```python
from build123d import *

# Parameters (mm, degrees)
F0_W     = 75
F0_H     = 70
F0_R     = 5
F0_R_2   = 2
F1_DEPTH = 2
F2_DEPTH = 7


with BuildPart() as f1:
    # F0 (on Top) → F1 (new body)
    with BuildSketch(Plane.XY):
        with Locations((4.717057, 0)):
            Rectangle(F0_W, F0_H)
        with Locations((4.717057, 0)):
            Circle(F0_R, mode=Mode.SUBTRACT)
        with Locations((34.717057, 0)):
            Circle(F0_R_2, mode=Mode.SUBTRACT)
    extrude(amount=F1_DEPTH)

    # F0 (on Top) → F2 (join)
    with BuildSketch(Plane.XY):
        with Locations((4.717057, 0)):
            Circle(F0_R)
        with Locations((34.717057, 0)):
            Circle(F0_R_2)
    extrude(amount=F2_DEPTH)


solid = f1.part
```
Can you work these out from the model? Positions are in its coordinate system, mm. A direction names the side the tool comes from. Give positions to 0.01 mm unless a question says otherwise; leave off trailing zeros. Loops run counter-clockwise (first coordinate to the right, second up) from the corner with the lowest first, then second, coordinate; pieces in that order, holes last. Notation, with made-up numbers: M 3,28.5 L 10,28.5 A14 ccw 10,32.5 Z; hole C 80.25,-10.75 d3. An arc over 180 degrees is marked long. One line per question, with ' | ' between items. Start each with the question number.
Q1. If I drill on line 1 (Z direction, x = 20, y = -20.5); line 2 (Y direction, x = 1.5, z = 6.75); line 3 (Y direction, x = 34, z = 4.25), over which ranges is the centre line in solid material (lowest first)? Write a range as from..to.
Q2. If we section it at A-A (z = 4.75): Please give me the cut outline in (x, y).
Q3. If we section it at B-B (y = 0): Please give me the cut outline in (x, z), plus the area to 3 significant figures.
Q4. For pin 1 Ø1 at (x, y) = (30, 24) entering from +Z; pin 2 Ø1 at (x, z) = (5.5, 4.5) entering from -Y, each with a flat end and sliding along its axis, tell me the tip position at first contact or that it passes through.
Q5. If we section it at D-D (y = 7): Please give me the cut outline in (x, z), plus the area to 3 significant figures.
Q6. If we section it at C-C (x = 1): Please give me the cut outline in (y, z), plus the area to 3 significant figures.
Q7. If we mould it in two halves opening along X, with no side actions, what happens to faces 1 (the flat face through (4, -35, 1)), 2 (the cylindrical face through (9.486, 1.502, 4.465)), 3 (the flat face through (-32.783, 0, 1))? For each: +X half, -X half, draft (parallel to the pull), parting line (faces both ways), or undercut.
Q8. For faces 4 (the cylindrical face through (32.72, 0.09, 4.46)), 5 (the flat face through (4, 35, 1)), which set-ups out of +Z, -Z, +X, -X, +Y, -Y let a thin tool reach every point of the face, with its end or its side?
Computed:
1) line 1: z = 0..2 | line 2: y = -3.83..3.83 | line 3: y = -1.87..1.87
2) outline: C 4.72,0 d10; C 34.72,0 d4
3) outline: M -32.78,0 L 42.22,0 L 42.22,2 L 36.72,2 L 36.72,7 L 32.72,7 L 32.72,2 L 9.72,2 L 9.72,7 L -0.28,7 L -0.28,2 L -32.78,2 Z | area: 220 mm²
4) pin 1: stops at z = 2 | pin 2: stops at y = -4.99
5) outline: M -32.78,0 L 42.22,0 L 42.22,2 L -32.78,2 Z | area: 150 mm²
6) outline: M -35,0 L 35,0 L 35,2 L 3.34,2 L 3.34,7 L -3.34,7 L -3.34,2 L -35,2 Z | area: 173 mm²
7) face 1: draft | face 2: undercut | face 3: -X half
8) face 4: +Z | face 5: +Z, -Z, +X, -X, +Y
